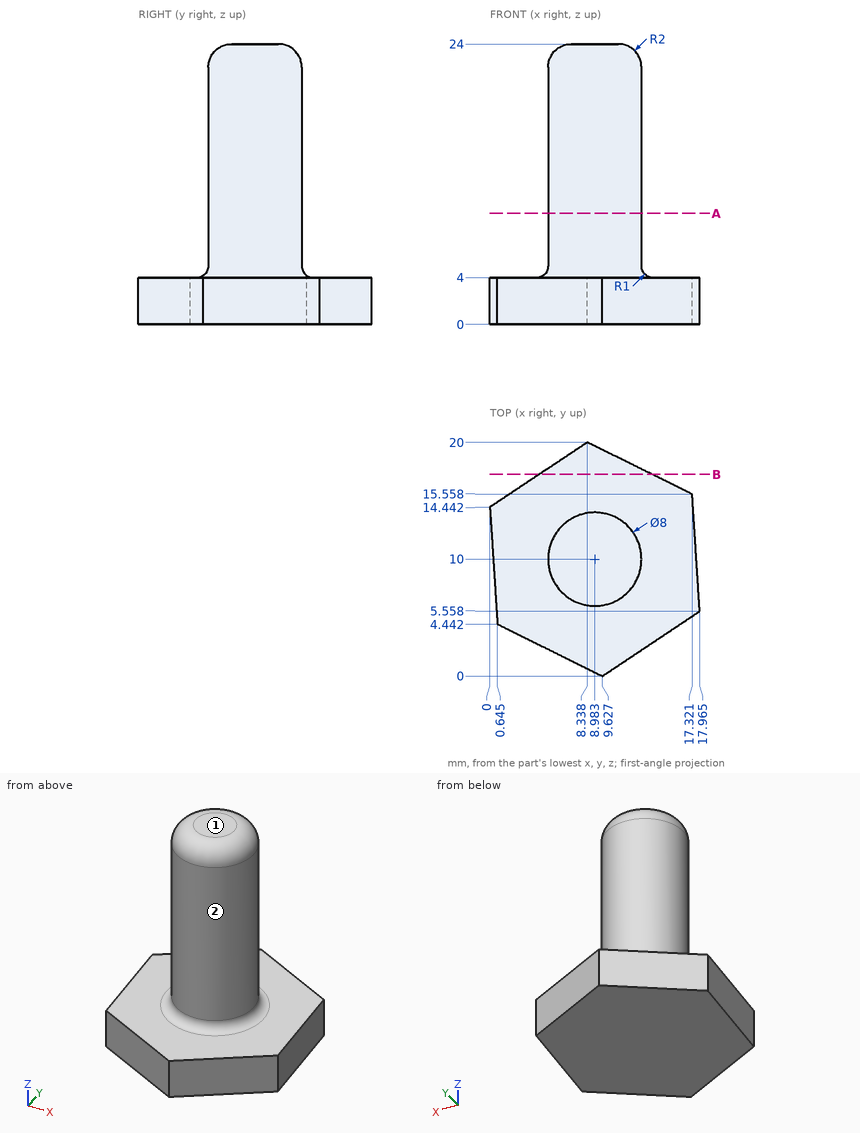
Verification items for this drawing (mm, ordinates from the low corner). A direction names the side the tool comes from. Round coordinates to 2 decimals unless told otherwise and drop trailing zeros. Order: outer loops, then holes, each group sorted by start corner. A loop starts at its lowest first (then second) coordinate and runs counter-clockwise, first axis right, second up. Notation, with made-up numbers: M 37.25,-8 L 51.25,-8 A30 cw 51.25,18 Z; hole C 59,88 d2. An arc over 180 degrees is marked long. Answer in a Markdown table with one row per item. Add a question column.
Item 1: Set-up check for the marked faces 1 and 2: record each of +Z, -Z, +X, -X, +Y, -Y from which the full face is reachable in a straight line by a thin tool's end or side.
Item 2: Sectioned sample at B-B, the plane y = 17.25. Enter the section's corners in (x, z).
Item 3: Depth check by flat-ended pin: pin 1 Ø4 at (x, z) = (12.5, 4.5) entering from -Y (1 decimal); pin 2 Ø1 at (x, y) = (2, 17) entering from -Z; pin 3 Ø3 at (x, z) = (11.5, 20) entering from +Y; pin 4 Ø8 at (y, z) = (16, 14) entering from +X. Enter the tip coordinate at first touch or a pass-through.
Item 4: Sectioned sample at A-A, the plane z = 9.5. Enter the section's corners in (x, y).
Item 5: Material ranges on L1, parallel to Z at x = 10.5, y = 17.5; L2, parallel to X at y = 5, z = 3.5 (1 decimal); L3, parallel to Y at x = 7.5, z = 17 (1 decimal), recorded low to high. Write a range as [from, to].
Filled in:
| question | item | result |
|---|---|---|
| 1 | face 1 | +Z, +X, -X, +Y, -Y |
| 1 | face 2 | +Z |
| 2 | outline | M 4.21,0 L 13.9,0 L 13.9,4 L 4.21,4 Z |
| 3 | pin 1 | stops at y = 0.6 |
| 3 | pin 2 | passes through |
| 3 | pin 3 | stops at y = 13.87 |
| 3 | pin 4 | stops at x = 12.45 |
| 4 | outline | C 8.98,10 d8 |
| 5 | L1 | z = [0, 4] |
| 5 | L2 | x = [0.6, 17.1] |
| 5 | L3 | y = [6.3, 13.7] |
